Geometry check sheet. Reference: the model listing, model coordinates, mm. Face numbers are marked on the shaded views. A direction names the side the tool comes from. Round coordinates to 2 decimals unless told otherwise and drop trailing zeros. Write each loop counter-clockwise with the first axis right and the second up, starting at its lowest first coordinate (ties: lowest second). Pieces come first, ordered by that corner, then holes. Notation, with made-up numbers: M 45.25,28.5 L 74.25,28.5 A6 ccw 74.25,32.5 Z; hole C 82,19.25 d2. An arc over 180 degrees is marked long. Put each result on its own line as item: value. Start each with the question number.
(1) Mould release check, pull along Y, two halves, no side actions. Record for the marked faces 1, 2, 3 and 4: pulls with the +Y half, pulls with the -Y half, needs draft (parallel to the pull), parting line crosses it, or undercut.
(2) Gauge pin test, flat ends, axial feed: pin 1 (3 mm diameter, centred on x = 54.5, z = 4, fed in from -Y); pin 2 (1 mm diameter, centred on y = 31, z = 6, fed in from -X); pin 3 (5 mm diameter, centred on y = 42, z = 7.5, fed in from -X). Record the tip position at first contact, or that the pin passes through.
(3) Section check A-A on x = 44.5. Record the cut outline in (y, z).
(4) Tool access check on the marked faces 5, 6, 7, 8 and 9. Record the directions out of +Z, -Z, +X, -X, +Y, -Y that give a thin tool (end or side, any length) a straight path to the whole face; none if there is none.
(5) Material ranges on probe 1 along Y at (x, z) = (54, 1.75); probe 2 along Y at (x, z) = (42.5, 9.5); probe 3 along X at (y, z) = (52, 9.5), recorded low to high.
(6) Section check B-B on x = 21. Record the cut outline in (y, z), then the cut area to 3 significant figures.
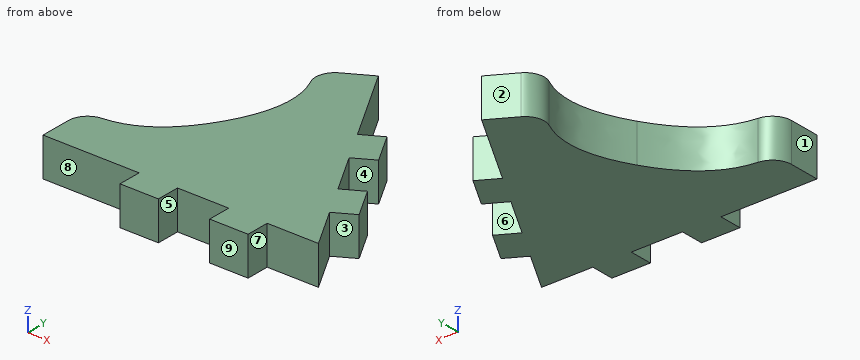
from build123d import *

# Parameters (mm, degrees)
BOSS_EXTRUDE1_DEPTH = 10
FILLET1_R           = 5


with BuildPart() as part:
    # Sketch1 → Boss-Extrude1 (new body)
    with BuildSketch(Plane.XY):
        with BuildLine():
            Line((36.66666666, -6), (36.66666666, 0))
            Line((36.66666666, 0), (23.33333333, 0))
            Line((23.33333333, 0), (23.33333333, -6))
            Line((23.33333333, -6), (13.33333333, -6))
            Line((13.33333333, -6), (13.33333333, 0))
            Line((13.33333333, 0), (-11.66666667, 0))
            Line((-11.66666667, 0), (-11.66666667, 13))
            add(Edge.make_bspline(
                [(-11.66666667, 13), (-1.66449563, 11.980359681), (6.23568211, 16.877469798), (12.368602782, 27.5)],
                knots=[0, 0, 0, 0, 1, 1, 1, 1], degree=3))
            add(Edge.make_bspline(
                [(12.908336411, 55.565153932), (18.792456349, 47.412839878), (18.501523453, 38.122530202), (12.368602782, 27.5)],
                knots=[0, 0, 0, 0, 1, 1, 1, 1], degree=3))
            Line((12.908336411, 55.565153932), (24.16666666, 62.065153932))
            Line((24.16666666, 62.065153932), (36.66666666, 40.414518838))
            Line((36.66666666, 40.414518838), (41.862819083, 43.414518838))
            Line((41.862819083, 43.414518838), (46.862819083, 34.7542648))
            Line((46.862819083, 34.7542648), (41.66666666, 31.7542648))
            Line((41.66666666, 31.7542648), (48.333333325, 20.207259419))
            Line((48.333333325, 20.207259419), (53.529485748, 23.207259419))
            Line((53.529485748, 23.207259419), (58.529485748, 14.547005381))
            Line((58.529485748, 14.547005381), (53.333333325, 11.547005381))
            Line((53.333333325, 11.547005381), (59.99999999, 0))
            Line((59.99999999, 0), (46.66666666, 0))
            Line((46.66666666, 0), (46.66666666, -6))
            Line((46.66666666, -6), (36.66666666, -6))
        make_face()
    extrude(amount=BOSS_EXTRUDE1_DEPTH)

    # Fillet1
    fillet1_edges = [part.edges().sort_by_distance(p)[0] for p in [
        (-11.66666667, 13, 5),
        (12.908336411, 55.565153932, 5),
    ]]
    fillet(fillet1_edges, radius=FILLET1_R)


solid = part.part
Answers follow:
1. face 1: needs draft
1. face 2: pulls with the +Y half
1. face 3: undercut
1. face 4: undercut
2. pin 1: stops at y = 0
2. pin 2: stops at x = 13.96
2. pin 3: stops at x = 16.88
3. outline: M -6,0 L 26.85,0 L 26.85,10 L -6,10 Z; M 33.39,0 L 38.85,0 L 38.85,10 L 33.39,10 Z
4. face 5: +Z, -Z, -Y
4. face 6: +Z, -Z, +Y
4. face 7: +Z, -Z, +X, -Y
4. face 8: +Z, -Z, -X, -Y
4. face 9: +Z, -Z, +X, -X, -Y
5. probe 1: y = 0 to 10.39, 11.93 to 22.39
5. probe 2: y = -6 to 30.31, 32.24 to 42.31
5. probe 3: x = 15.07 to 29.98
6. outline: M -6,0 L 60.24,0 L 60.24,10 L -6,10 Z
6. area: 662 mm^2
